from build123d import *

# Parameters (mm, degrees)
F1_DEPTH = 5
F2_R     = 8
F3_DEPTH = 3


# Not quite as in the source:
# - a fillet or chamfer that OpenCascade refuses, or shapes differently, is made with other operations: its cross-section is extruded or revolved along the edge and cut away or added


with BuildPart() as f1:
    # F0 (on Top) → F1 (new body)
    with BuildSketch(Plane.XY):
        Polygon((4.5920703038, -0.2481590048), (2.8108349475, 3.333349142), (-1.1814597696, 3.5815081468), (-3.3925191305, 0.2481590048), (-1.6112837742, -3.333349142), (2.3810109429, -3.5815081468), align=None)
    extrude(amount=F1_DEPTH)

    # F2 (on face) → F3 (join)
    with BuildSketch(Plane(origin=(0, 0, 0), x_dir=(1, 0, 0), z_dir=(0, 0, -1))):
        with Locations((0.5997755867, 0)):
            Circle(F2_R)
        Polygon((2.8108349475, -3.333349142), (-1.1814597696, -3.5815081468), (-3.3925191305, -0.2481590048), (-1.6112837742, 3.333349142), (2.3810109429, 3.5815081468), (4.5920703038, 0.2481590048), align=None, mode=Mode.SUBTRACT)
        Polygon((-3.3925191305, -0.2481590048), (-1.1814597696, -3.5815081468), (2.8108349475, -3.333349142), (4.5920703038, 0.2481590048), (2.3810109429, 3.5815081468), (-1.6112837742, 3.333349142), align=None)
    extrude(amount=F3_DEPTH)

    # F4: fillet of radius 5 on 1 edges, made by hand

    # F4_s1 → F4_t2 (revolve, cut)
    with BuildSketch(Plane.XZ):
        with BuildLine():
            ThreePointArc((8.5997755867, 0), (6.7558126792, -2.1833001327), (4.0171998917, -3))
            Line((4.0171998917, -3), (8.5997755867, -3))
            Line((8.5997755867, -3), (8.5997755867, 0))
        make_face()
    revolve(axis=Axis((0.5997755867, 0, -3), (0, 0, -1)), mode=Mode.SUBTRACT)


solid = f1.part
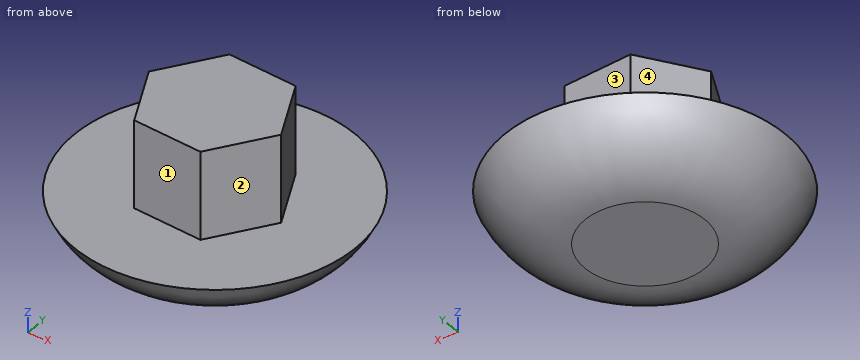
Geometry: final body of the model. Coordinates: model frame, mm. Face numbers are marked on the shaded views. A direction names the side the tool comes from. Coordinates: 2 decimals unless noted, no trailing zeros. Loops run counter-clockwise (first coordinate to the right, second up) from the corner with the lowest first, then second, coordinate; pieces in that order, holes last. Notation, with made-up numbers: (9.5, 72) - (57.5, 72) arc R22 ccw to (57.5, 84) - close; hole circle Ø9 at (62, 77). An arc over 180 degrees is marked (long way). Put each result on its own line as item: value. Start each with the question number.
Q1. Pin query (flat end, axial travel): pin 1 Ø1.5 at (y, z) = (2, -0.5) entering from +X; pin 2 Ø1 at (y, z) = (-3.5, 4) entering from -X; pin 3 Ø1 at (y, z) = (0.5, 1) entering from -X; pin 4 Ø1 at (y, z) = (-5.5, 3) entering from +X. Return the tip coordinate at first contact, or that it passes through.
Q2. Line query: line 1 (Y direction, x = 4.75, z = -0.25); line 2 (Y direction, x = 4, z = 2.5); line 3 (Z direction, x = -5, y = 3). Output: solid intervals per line, ascending.
Q3. Cut plane A-A, the plane z = 3.25. Return loops of the section in (x, y).
Q4. Set-up query: the marked faces 1, 2, 3 and 4. Return all of +Z, -Z, +X, -X, +Y, -Y with unobstructed straight access to the full face (end or side cutting, diameter ignored); none if empty.
Filled sheet:
1. pin 1: x = 8.47
1. pin 2: x = -1.78
1. pin 3: x = -3.39
1. pin 4: through
2. line 1: -6.7 to 6.7
2. line 2: -1.14 to 0.94
2. line 3: -2.05 to 0
3. outline: (-3.39, 0.25) - (-1.61, -3.33) - (2.38, -3.58) - (4.59, -0.25) - (2.81, 3.33) - (-1.18, 3.58) - close
4. face 1: +Z, -X, -Y
4. face 2: +Z, +X, -Y
4. face 3: +Z, +X, +Y
4. face 4: +Z, -X, +Y
